```python
from build123d import *

# Parameters (mm, degrees)
BOSS_EXTRU_1_DEPTH = 40
D_GAGEMENT_M41_D   = 4.5
D_GAGEMENT_M42_D   = 4.5


with BuildPart() as part:
    # Esquisse1 → Boss.-Extru.1 (new body)
    with BuildSketch(Plane.XY):
        Polygon((0, 36), (0, 0), (36, 0), (36, -4), (-4, -4), (-4, 36), align=None)
    extrude(amount=BOSS_EXTRU_1_DEPTH)

    # Dégagement M41 (through all)
    with Locations(Plane(origin=(0, 0, 0), x_dir=(1, 0, 0), z_dir=(0, 1, 0))):
        with Locations((18, -20)):
            Hole(D_GAGEMENT_M41_D / 2)

    # Dégagement M42 (through all)
    with Locations(Plane(origin=(0, 0, 0), x_dir=(0, 0, -1), z_dir=(1, 0, 0))):
        with Locations((-20, 16)):
            Hole(D_GAGEMENT_M42_D / 2)


solid = part.part
```
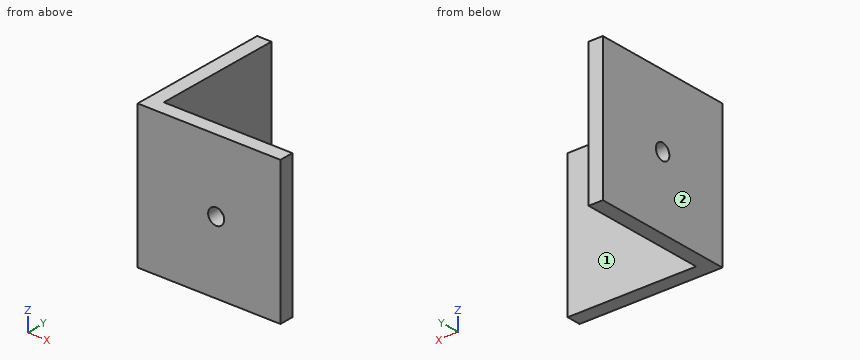
Could you check a few things on this model? Use its own coordinates, in mm. Face numbers are marked on the shaded views. A direction names the side the tool comes from. Coordinates: 2 decimals unless noted, no trailing zeros. Write each loop counter-clockwise with the first axis right and the second up, starting at its lowest first coordinate (ties: lowest second). Pieces come first, ordered by that corner, then holes. Notation, with made-up numbers: (78, 51.25) -> (123, 51.25) arc R9 ccw to (123, 68.25) -> close; hole circle Ø7 at (-18.75, 31). An arc over 180 degrees is marked (long way). One line per question, with ' | ' between items. Start each with the question number.
1. Will these pins go through, and if not, where does the flat tip stop? P1, Ø4, axis at y = 16, z = 20, coming from the +X side; P2, Ø3, axis at x = 21, z = 4, coming from the +Y side; P3, Ø11, axis at y = 17, z = 19.5, coming from the +X side.
2. For the marked faces 1 and 2, which set-ups out of +Z, -Z, +X, -X, +Y, -Y let a thin tool reach every point of the face, with its end or its side?
3. If we section it at D-D (z = 28.5): Please give me the cut outline in (x, y).
4. If we section it at A-A (x = 18): Please give me the cut outline in (y, z), and give its area (3 significant figures).
5. If we section it at C-C (z = 20): Please give me the cut outline in (x, y).
6. Please list where these lines run through material, in increasing order: line 1 along Z through (x, y) = (18, -1.85); line 2 along X through (y, z) = (-2.4, 20); line 3 along Y through (x, z) = (6, 2.5).
Return value:
1) P1: passes through | P2: stops at y = 0 | P3: stops at x = 0
2) face 1: +Z, -Z, +X, +Y | face 2: +Z, -Z, -X, +Y, -Y
3) outline: (-4, -4) -> (36, -4) -> (36, 0) -> (0, 0) -> (0, 36) -> (-4, 36) -> close
4) outline: (-4, 0) -> (0, 0) -> (0, 17.75) -> (-4, 17.75) -> close; (-4, 22.25) -> (0, 22.25) -> (0, 40) -> (-4, 40) -> close | area: 142 mm²
5) outline: (-4, -4) -> (15.75, -4) -> (15.75, 0) -> (0, 0) -> (0, 13.75) -> (-4, 13.75) -> close; (-4, 18.25) -> (0, 18.25) -> (0, 36) -> (-4, 36) -> close; (20.25, -4) -> (36, -4) -> (36, 0) -> (20.25, 0) -> close
6) line 1: z = 0 to 17.75, 22.25 to 40 | line 2: x = -4 to 15.75, 20.25 to 36 | line 3: y = -4 to 0
